Could you check a few things on this model? Use its own coordinates, in mm. Round coordinates to 2 decimals unless told otherwise and drop trailing zeros. Loops run counter-clockwise (first coordinate to the right, second up) from the corner with the lowest first, then second, coordinate; pieces in that order, holes last. Notation, with made-up numbers: (-3.5, 55) -> (32.5, 55) arc R19 cw to (32.5, 89) -> close; hole circle Ø10 at (-17.5, 6). An arc over 180 degrees is marked (long way). Write each question's results on one line, items separated by ' | '.
from build123d import *

# Parameters (mm, degrees)
SKETCH1_R           = 15.027499291
BOSS_EXTRUDE1_DEPTH = 6.096
SKETCH2_R           = 15.027499291
BOSS_EXTRUDE2_DEPTH = 1.778
CHAMFER1_SIZE       = 0.381
SKETCH3_R           = 6.35
BOSS_EXTRUDE3_DEPTH = 3.048
CHAMFER2_SIZE       = 0.381


with BuildPart() as part:
    # Sketch1 → Boss-Extrude1 (new body)
    with BuildSketch(Plane(origin=(0, 0, 0), x_dir=(1, 0, 0), z_dir=(0, 1, 0))):
        Circle(SKETCH1_R)
        with BuildLine():
            ThreePointArc((-9.464927768, -3.0607), (-7.033944205, -7.033944205), (-3.0607, -9.464927768))
            Line((-3.0607, -9.464927768), (-3.0607, -10.984341946))
            ThreePointArc((-3.0607, -10.984341946), (-2.896474772, -11.380816718), (-2.5, -11.545041946))
            Line((-2.5, -11.545041946), (2.5, -11.545041946))
            ThreePointArc((2.5, -11.545041946), (2.896474772, -11.380816718), (3.0607, -10.984341946))
            Line((3.0607, -10.984341946), (3.0607, -9.464927768))
            ThreePointArc((3.0607, -9.464927768), (7.033944205, -7.033944205), (9.464927768, -3.0607))
            Line((9.464927768, -3.0607), (10.984341946, -3.0607))
            ThreePointArc((10.984341946, -3.0607), (11.380816718, -2.896474772), (11.545041946, -2.5))
            Line((11.545041946, -2.5), (11.545041946, 2.5))
            ThreePointArc((11.545041946, 2.5), (11.380816718, 2.896474772), (10.984341946, 3.0607))
            Line((10.984341946, 3.0607), (9.464927768, 3.0607))
            ThreePointArc((9.464927768, 3.0607), (7.033944205, 7.033944205), (3.0607, 9.464927768))
            Line((3.0607, 9.464927768), (3.0607, 10.984341946))
            ThreePointArc((3.0607, 10.984341946), (2.896474772, 11.380816718), (2.5, 11.545041946))
            Line((2.5, 11.545041946), (-2.5, 11.545041946))
            ThreePointArc((-2.5, 11.545041946), (-2.896474772, 11.380816718), (-3.0607, 10.984341946))
            Line((-3.0607, 10.984341946), (-3.0607, 9.464927768))
            ThreePointArc((-3.0607, 9.464927768), (-7.033944205, 7.033944205), (-9.464927768, 3.0607))
            Line((-9.464927768, 3.0607), (-10.984341946, 3.0607))
            ThreePointArc((-10.984341946, 3.0607), (-11.380816718, 2.896474772), (-11.545041946, 2.5))
            Line((-11.545041946, 2.5), (-11.545041946, -2.5))
            ThreePointArc((-11.545041946, -2.5), (-11.380816718, -2.896474772), (-10.984341946, -3.0607))
            Line((-10.984341946, -3.0607), (-9.464927768, -3.0607))
        make_face(mode=Mode.SUBTRACT)
    extrude(amount=BOSS_EXTRUDE1_DEPTH)

    # Sketch2 → Boss-Extrude2 (add)
    with BuildSketch(Plane(origin=(0, 6.096, 0), x_dir=(1, 0, 0), z_dir=(0, 1, 0))):
        Circle(SKETCH2_R)
    extrude(amount=BOSS_EXTRUDE2_DEPTH)

    # Chamfer1
    chamfer1_edges = [part.edges().sort_by_distance(p)[0] for p in [
        (-3.0607, 0, 10.224634857),
        (-2.896474772, 0, 11.380816718),
        (0, 0, 11.545041946),
        (2.896474772, 0, 11.380816718),
        (3.0607, 0, 10.224634857),
        (10.224634857, 0, 3.0607),
        (11.380816718, 0, 2.896474772),
        (11.545041946, 0, 0),
        (11.380816718, 0, -2.896474772),
        (10.224634857, 0, -3.0607),
        (3.0607, 0, -10.224634857),
        (2.896474772, 0, -11.380816718),
        (0, 0, -11.545041946),
        (-2.896474772, 0, -11.380816718),
        (-3.0607, 0, -10.224634857),
        (-10.224634857, 0, -3.0607),
        (-11.380816718, 0, -2.896474772),
        (-11.545041946, 0, 0),
        (-11.380816718, 0, 2.896474772),
        (-10.224634857, 0, 3.0607),
    ]]
    chamfer(chamfer1_edges, length=CHAMFER1_SIZE)

    # Sketch3 → Boss-Extrude3 (add)
    with BuildSketch(Plane(origin=(0, 7.874, 0), x_dir=(1, 0, 0), z_dir=(0, 1, 0))):
        Circle(SKETCH3_R)
    extrude(amount=BOSS_EXTRUDE3_DEPTH)

    # Chamfer2
    chamfer2_edges = [part.edges().sort_by_distance(p)[0] for p in [
        (-6.35, 10.922, 0),
    ]]
    chamfer(chamfer2_edges, length=CHAMFER2_SIZE)


solid = part.part
1) I want a section at D-D, the plane y = 7.25. Write out the boundary of the cut face in (x, z) (1 decimal), plus the area to 3 significant figures.
Model answer:
outline: circle Ø30.1 at (0, 0) | area: 709 mm2
2) I want a section at B-B, the plane z = 0. Write out the boundary of the cut face in (x, y), plus the area to 3 significant figures.
Model answer:
outline: (-15.03, 0) -> (-11.93, 0) -> (-11.55, 0.38) -> (-11.55, 6.1) -> (11.55, 6.1) -> (11.55, 0.38) -> (11.93, 0) -> (15.03, 0) -> (15.03, 7.87) -> (6.35, 7.87) -> (6.35, 10.54) -> (5.97, 10.92) -> (-5.97, 10.92) -> (-6.35, 10.54) -> (-6.35, 7.87) -> (-15.03, 7.87) -> close | area: 134 mm2
3) I need wall thicknesses on line 1 (Y direction, x = 0.5, z = 7.5); line 2 (Y direction, x = 3, z = 1.5); line 3 (X direction, y = 5, z = -1). Which ranges of each line are inside material? Lowest first, please.
Model answer:
line 1: y = 6.1 to 7.87 | line 2: y = 6.1 to 10.92 | line 3: x = -14.99 to -11.55, 11.55 to 14.99
4) I'm going to push flat-ended pins straight in: pin 1 (0.8 mm diameter, centred on y = 2, z = 10.5, fed in from +X); pin 2 (4 mm diameter, centred on x = 0.5, y = 3.5, fed in from -Z); pin 3 (7 mm diameter, centred on x = -1, z = 2.5, fed in from -Y); pin 4 (3 mm diameter, centred on x = -7, y = 2.5, fed in from +Z). Where does each tip first touch, or does it pass through?
Model answer:
pin 1: stops at x = 11.13 | pin 2: stops at z = -15.03 | pin 3: stops at y = 6.1 | pin 4: stops at z = 13.98
5) I want a section at A-A, the plane y = 5.25. Write out the boundary of the cut face in (x, z) (1 decimal).
Model answer:
outline: circle Ø30.1 at (0, 0); hole (-11.5, -2.5) arc R0.6 ccw to (-11, -3.1) -> (-9.5, -3.1) arc R9.9 ccw to (-3.1, -9.5) -> (-3.1, -11) arc R0.6 ccw to (-2.5, -11.5) -> (2.5, -11.5) arc R0.6 ccw to (3.1, -11) -> (3.1, -9.5) arc R9.9 ccw to (9.5, -3.1) -> (11, -3.1) arc R0.6 ccw to (11.5, -2.5) -> (11.5, 2.5) arc R0.6 ccw to (11, 3.1) -> (9.5, 3.1) arc R9.9 ccw to (3.1, 9.5) -> (3.1, 11) arc R0.6 ccw to (2.5, 11.5) -> (-2.5, 11.5) arc R0.6 ccw to (-3.1, 11) -> (-3.1, 9.5) arc R9.9 ccw to (-9.5, 3.1) -> (-11, 3.1) arc R0.6 ccw to (-11.5, 2.5) -> close
6) I want a section at C-C, the plane x = -7. Write out the boundary of the cut face in (y, z), plus the area to 3 significant figures.
Model answer:
outline: (0, -13.3) -> (7.87, -13.3) -> (7.87, 13.3) -> (0, 13.3) -> (0, 7.07) -> (6.1, 7.07) -> (6.1, -7.07) -> (0, -7.07) -> close | area: 123 mm2
